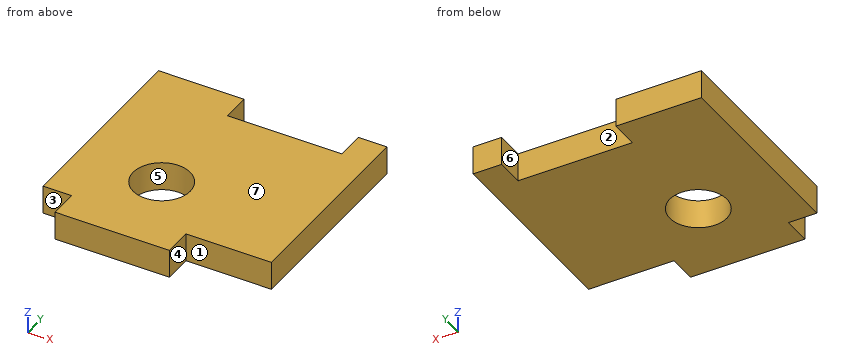
```python
from build123d import *

# Parameters (mm, degrees)
F0_W     = 3.175
F0_H     = 3.175
F0_W_2   = 9.525
F0_R     = 3.175
F1_DEPTH = 3.175


with BuildPart() as f1:
    # F0 (on Top) → F1 (new body)
    with BuildSketch(Plane.XY):
        Polygon((9.525, 9.525), (9.525, -9.525), (15.875, -9.525), (15.875, 9.525), (12.7, 9.525), align=None)
        with Locations((14.2875, 11.1125)):
            Rectangle(F0_W, F0_H)
        with Locations((-4.7625, 11.1125)):
            Rectangle(F0_W_2, F0_H)
        Polygon((6.35, -9.525), (9.525, -9.525), (9.525, 9.525), (0, 9.525), (-9.525, 9.525), (-9.525, -9.525), (-6.35, -9.525), (-6.35, -12.7), (6.35, -12.7), align=None)
        with Locations((0, -3.175)):
            Circle(F0_R, mode=Mode.SUBTRACT)
    extrude(amount=F1_DEPTH)


solid = f1.part
```
Verification items for the finished model (mm, model axes). Face numbers are marked on the shaded views. A direction names the side the tool comes from. Coordinates: 2 decimals unless noted, no trailing zeros. Loops run counter-clockwise (first coordinate to the right, second up) from the corner with the lowest first, then second, coordinate; pieces in that order, holes last. Notation, with made-up numbers: (15.25, -2.5) -> (26.25, -2.5) arc R12 cw to (26.25, 7.5) -> close; hole circle Ø9 at (65, 41). An arc over 180 degrees is marked (long way). Answer in a Markdown table with one row per item. Add a question column.
1. Section check D-D, the plane x = 13. Enter the section's corners in (y, z) (3 decimals), then the cut area to 3 significant figures.
2. Section check A-A, the plane z = 0.55. Enter the section's corners in (x, y) (3 decimals), then the cut area to 3 significant figures.
3. Section check B-B, the plane y = 10. Enter the section's corners in (x, z) (3 decimals), then the cut area to 3 significant figures.
4. Depth check by flat-ended pin: P1, Ø1.6, axis at x = -8, z = 1, coming from the -Y side (3 decimals); P2, Ø1.6, axis at y = -11, z = 1.5, coming from the -X side; P3, Ø1, axis at y = -10.5, z = 2, coming from the +X side; P4, Ø5.5, axis at x = 0, y = -3.175, coming from the +Z side. Enter the tip coordinate at first touch or a pass-through.
5. Access from +Z, -Z, +X, -X, +Y, -Y to the whole of each face (thin tool, end or side, straight path). Record for the marked faces 1, 2 and 3.
6. Draft check along X on the marked faces 4, 5, 6 and 7. Enter one of: +X half, -X half, draft (parallel to the pull), parting line (faces both ways), or undercut.
7. Section check C-C, the plane x = 1.5. Enter the section's corners in (y, z) (3 decimals), then the cut area to 3 significant figures.
8. Material ranges on probe 1 along X at (y, z) = (-10.75, 1); probe 2 along Y at (x, z) = (13.75, 0.45) (3 decimals); probe 3 along Y at (x, z) = (8.25, 2.2) (3 decimals), recorded low to high. Write a range as [from, to].
Derived:
| question | item | result |
|---|---|---|
| 1 | outline | (-9.525, 0) -> (12.7, 0) -> (12.7, 3.175) -> (-9.525, 3.175) -> close |
| 1 | area | 70.6 mm² |
| 2 | outline | (-9.525, -9.525) -> (-6.35, -9.525) -> (-6.35, -12.7) -> (6.35, -12.7) -> (6.35, -9.525) -> (15.875, -9.525) -> (15.875, 12.7) -> (12.7, 12.7) -> (12.7, 9.525) -> (0, 9.525) -> (0, 12.7) -> (-9.525, 12.7) -> close; hole circle Ø6.35 at (0, -3.175) |
| 2 | area | 533 mm² |
| 3 | outline | (-9.525, 0) -> (0, 0) -> (0, 3.175) -> (-9.525, 3.175) -> close; (12.7, 0) -> (15.875, 0) -> (15.875, 3.175) -> (12.7, 3.175) -> close |
| 3 | area | 40.3 mm² |
| 4 | P1 | stops at y = -9.525 |
| 4 | P2 | stops at x = -6.35 |
| 4 | P3 | stops at x = 6.35 |
| 4 | P4 | passes through |
| 5 | face 1 | +Z, -Z, +X, -Y |
| 5 | face 2 | +Z, -Z, +Y |
| 5 | face 3 | +Z, -Z, -X, -Y |
| 6 | face 4 | +X half |
| 6 | face 5 | undercut |
| 6 | face 6 | undercut |
| 6 | face 7 | draft |
| 7 | outline | (-12.7, 0) -> (-5.973, 0) -> (-5.973, 3.175) -> (-12.7, 3.175) -> close; (-0.377, 0) -> (9.525, 0) -> (9.525, 3.175) -> (-0.377, 3.175) -> close |
| 7 | area | 52.8 mm² |
| 8 | probe 1 | x = [-6.35, 6.35] |
| 8 | probe 2 | y = [-9.525, 12.7] |
| 8 | probe 3 | y = [-9.525, 9.525] |
